from build123d import *

# Parameters (mm, degrees)
SKETCH_R             = 8.5
SKETCH_R_2           = 7.15
PAD_DEPTH            = 11
REVOLUTION_FACE2_R   = 8.5
REVOLUTION_FACE2_R_2 = 7.15
PAD001_DEPTH         = 1


with BuildPart() as part:
    # Sketch → Pad (new body)
    with BuildSketch(Plane.XY):
        Circle(SKETCH_R)
        Circle(SKETCH_R_2, mode=Mode.SUBTRACT)
    extrude(amount=PAD_DEPTH)

    # Sketch001 → Revolution (revolve)
    with BuildSketch(Plane.XZ):
        Polygon((7.154231, 10.959348), (11.531741, 13.844253), (12.016494, 13.802702), (12.265796, 13.5811), (12.238096, 13.124048), (8.581674, 8.456569), align=None)
    revolve(axis=Axis((0, 0, 0), (0, 0, 1)))

    # Revolution Face2 → Pad001 (add)
    with BuildSketch(Plane(origin=(0, 0, 0), x_dir=(0, -1, 0), z_dir=(0, 0, -1))):
        Circle(REVOLUTION_FACE2_R)
        Circle(REVOLUTION_FACE2_R_2, mode=Mode.SUBTRACT)
    extrude(amount=PAD001_DEPTH)


solid = part.part
Work out the finished part from the listing and answer in its coordinate system (mm). Coordinates: 2 decimals unless noted, no trailing zeros. Write each loop counter-clockwise with the first axis right and the second up, starting at its lowest first coordinate (ties: lowest second). Pieces come first, ordered by that corner, then holes.
1. The part is cut by section A-A, the plane x = 0. Write down the section's boundary in (y, z).
Results list:
outline: (-12.27, 13.58) - (-12.24, 13.12) - (-8.58, 8.46) - (-8.5, 8.6) - (-8.5, -1) - (-7.15, -1) - (-7.15, 11) - (-7.22, 11) - (-11.53, 13.84) - (-12.02, 13.8) - close; (7.15, -1) - (8.5, -1) - (8.5, 8.6) - (8.58, 8.46) - (12.24, 13.12) - (12.27, 13.58) - (12.02, 13.8) - (11.53, 13.84) - (7.22, 11) - (7.15, 11) - close
2. For a pull along X with two mould halves and no side action, classify faces 1 (the conical face through (8.35, 2.63, 8.68)), 2 (the conical face through (-1.62, -7.31, 11.18)) as +X half, -X half, draft (parallel to the pull), parting line (faces both ways), or undercut.
Results list:
face 1: parting line
face 2: undercut
3. Flat-ended cylindrical pins translate along their axes: pin 1 (6 mm diameter, centred on x = -2, z = 7, fed in from +Y); pin 2 (2 mm diameter, centred on x = 0, z = 9, fed in from +Y); pin 3 (2 mm diameter, centred on x = 7, z = 12, fed in from -Y); pin 4 (8.5 mm diameter, centred on x = 0, y = 0, fed in from +Z). Find the tip coordinate at first contact, or state that the pin passes through.
Results list:
pin 1: stops at y = 9.64
pin 2: stops at y = 9.79
pin 3: stops at y = -10.13
pin 4: passes through
4. The part is cut by section C-C, the plane z = 2. Write down the section's boundary in (x, y).
Results list:
outline: circle Ø17 at (0, 0); hole circle Ø14.3 at (0, 0)
5. Consider line 1 along X through (y, z) = (0, -0.7); line 2 along Z through (x, y) = (-6, -4). Determine where each line is inside the solid, lowest interval first.
Results list:
line 1: x = -8.5 to -7.15, 7.15 to 8.5
line 2: z = -1 to 11
6. The part is cut by section D-D, the plane z = 10. Write down the section's boundary in (x, y).
Results list:
outline: circle Ø19.58 at (0, 0); hole circle Ø14.3 at (0, 0)
